Can you work these out from the drawing? Everything is in mm from the part's minimum corner. Coordinates: 2 decimals unless noted, no trailing zeros. Loops run counter-clockwise (first coordinate to the right, second up) from the corner with the lowest first, then second, coordinate; pieces in that order, holes last.
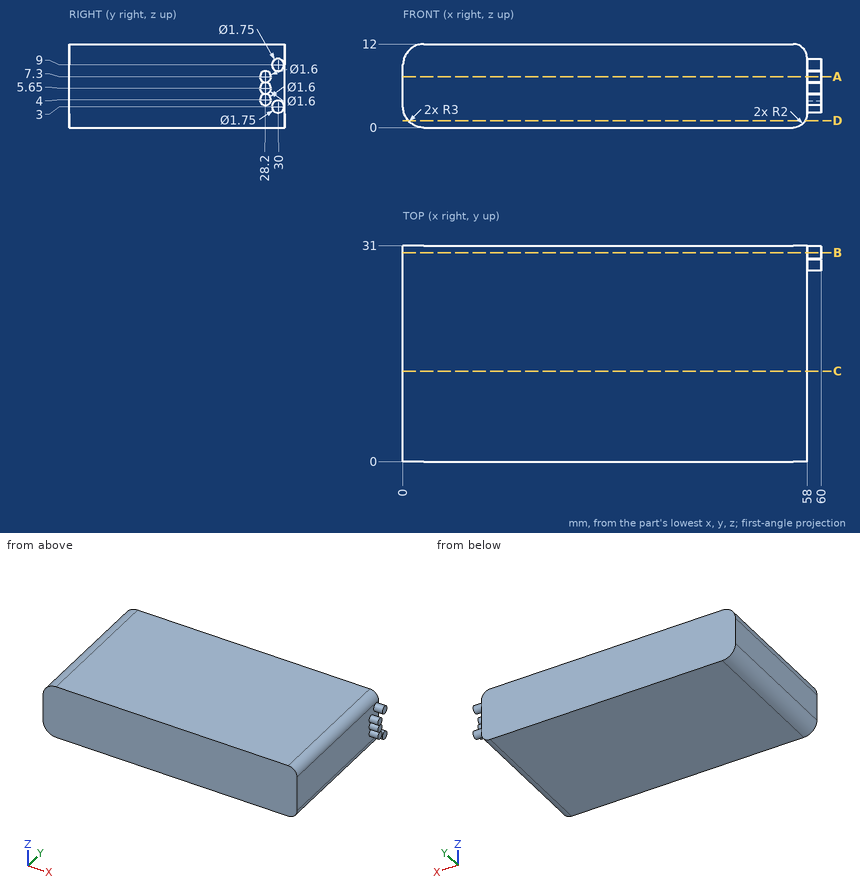
(1) Imagine slicing it at C-C, the plane y = 13. Write out the boundary of the cut face in (x, z).
Answers:
outline: (0, 3) arc R3 ccw to (3, 0) - (56, 0) arc R2 ccw to (58, 2) - (58, 10) arc R2 ccw to (56, 12) - (3, 12) arc R3 ccw to (0, 9) - close
(2) Imagine slicing it at B-B, the plane y = 30. Write out the boundary of the cut face in (x, z) (3 decimals), and give its area (3 significant figures).
Answers:
outline: (0, 3) arc R3 ccw to (3, 0) - (56, 0) arc R2 ccw to (58, 2) - (58, 2.125) - (60, 2.125) - (60, 3.875) - (58, 3.875) - (58, 8.125) - (60, 8.125) - (60, 9.875) - (58, 9.875) - (58, 10) arc R2 ccw to (56, 12) - (3, 12) arc R3 ccw to (0, 9) - close
area: 697 mm2
(3) For pin 1 (2 mm diameter, centred on x = 33, z = 7, fed in from -Y); pin 2 (6.5 mm diameter, centred on y = 8, z = 4.5, fed in from +X), each with a flat end and sliding along its axis, tell me the tip position at first contact or that it passes through.
Answers:
pin 1: stops at y = 0
pin 2: stops at x = 58
(4) Imagine slicing it at D-D, the plane z = 1. Write out the boundary of the cut face in (x, y), and give its area (3 significant figures).
Answers:
outline: (0.76, 0) - (57.73, 0) - (57.73, 31) - (0.76, 31) - close
area: 1,770 mm2
(5) Imagine slicing it at A-A, the plane z = 7.3. Write out the boundary of the cut face in (x, y), and give its area (3 significant figures).
Answers:
outline: (0, 0) - (58, 0) - (58, 27.4) - (60, 27.4) - (60, 29) - (58, 29) - (58, 31) - (0, 31) - close
area: 1,800 mm2
(6) I need wall thicknesses on probe 1 along X at (y, z) = (29.5, 6.25); probe 2 along X at (y, z) = (11, 9.75). Which ranges of each line are inside material? Lowest first, please.
Answers:
probe 1: x = 0 to 58
probe 2: x = 0.1 to 58
